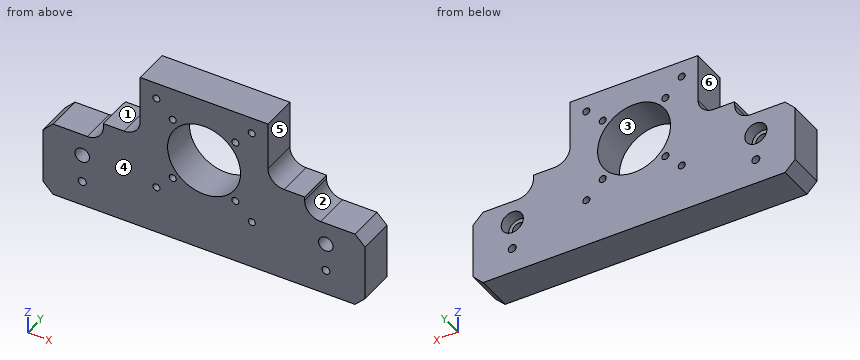
from build123d import *

# Parameters (mm, degrees)
F0_R           = 2
F0_W           = 63.5
F0_H           = 11.75
F0_R_2         = 1.75
F0_R_3         = 18.125
F1_DEPTH       = 18
F2_SIZE        = 5
F3_R           = 8
F4_D           = 7.2
F4_DEPTH       = 35
F4_CBORE_D     = 11
F4_CBORE_DEPTH = 6
F4_TIP         = 2.1630982285


with BuildPart() as f1:
    # F0 (on Front) → F1 (new body)
    with BuildSketch(Plane.XZ):
        Polygon((-80, -33.75), (80, -33.75), (80, 3.75), (50, 3.75), (50, 13.75), (31.75, 13.75), (31.75, -18), (-31.75, -18), (-31.75, 13.75), (-50, 13.75), (-50, 3.75), (-80, 3.75), align=None)
        with Locations((-60.5, -21.25)):
            Circle(F0_R, mode=Mode.SUBTRACT)
        with Locations((60.5, -21.25)):
            Circle(F0_R, mode=Mode.SUBTRACT)
        with Locations((0, 39.625)):
            Rectangle(F0_W, F0_H)
        with Locations((-23.6880771697, 37.4380771697)):
            Circle(F0_R_2, mode=Mode.SUBTRACT)
        with Locations((23.6880771697, 37.4380771697)):
            Circle(F0_R_2, mode=Mode.SUBTRACT)
        Polygon((31.75, 13.75), (31.75, 33.75), (-31.75, 33.75), (-31.75, 13.75), (-31.75, -18), (31.75, -18), align=None)
        with Locations((-23.6880771697, -9.9380771697)):
            Circle(F0_R_2, mode=Mode.SUBTRACT)
        with Locations((-15.5563491861, -1.8063491861)):
            Circle(F0_R_2, mode=Mode.SUBTRACT)
        with Locations((23.6880771697, -9.9380771697)):
            Circle(F0_R_2, mode=Mode.SUBTRACT)
        with Locations((15.5563491861, -1.8063491861)):
            Circle(F0_R_2, mode=Mode.SUBTRACT)
        with Locations((-15.5563491861, 29.3063491861)):
            Circle(F0_R_2, mode=Mode.SUBTRACT)
        with Locations((0, 13.75)):
            Circle(F0_R_3, mode=Mode.SUBTRACT)
        with Locations((15.5563491861, 29.3063491861)):
            Circle(F0_R_2, mode=Mode.SUBTRACT)
    extrude(amount=F1_DEPTH)

    # F2
    f2_edges = [f1.edges().sort_by_distance(p)[0] for p in [
        (-80, -9, -33.75),
        (80, -9, -33.75),
        (80, -9, 3.75),
        (-80, -9, 3.75),
    ]]
    chamfer(f2_edges, length=F2_SIZE)

    # F3
    f3_edges = [f1.edges().sort_by_distance(p)[0] for p in [
        (31.75, -9, 13.75),
        (-31.75, -9, 13.75),
        (50, -9, 3.75),
        (-50, -9, 3.75),
    ]]
    fillet(f3_edges, radius=F3_R)

    # F4
    with Locations(Plane(origin=(0, 0, 0), x_dir=(1, 0, 0), z_dir=(0, 1, 0))):
        with Locations((60.5, 7.25), (-60.5, 7.25)):
            CounterBoreHole(F4_D / 2, F4_CBORE_D / 2, F4_CBORE_DEPTH, depth=F4_DEPTH)
            with Locations((0, 0, -(F4_DEPTH + F4_TIP / 2))):  # 118° drill point
                Cone(0, F4_D / 2, F4_TIP, mode=Mode.SUBTRACT)


solid = f1.part
For this review, take the finished solid that the model builds, in its own axes (mm). Face numbers are marked on the shaded views. A direction names the side the tool comes from. Give positions to 0.01 mm unless a question says otherwise; leave off trailing zeros. Order: outer loops, then holes, each group sorted by start corner. A loop starts at its lowest first (then second) coordinate and runs counter-clockwise, first axis right, second up. Notation, with made-up numbers: (-17, 18.25) -> (25, 18.25) arc R22 cw to (25, 31.25) -> close; hole circle Ø2 at (55, 8). An arc over 180 degrees is marked (long way). Write item = value, one per line.
1) Insertion check: pin 1 (5 mm diameter, centred on x = 67.5, y = -8.5, fed in from +Z); pin 2 (2 mm diameter, centred on x = -15.56, z = -1.81, fed in from -Y); pin 3 (9 mm diameter, centred on x = -60.5, z = -7.25, fed in from +Y); pin 4 (8 mm diameter, centred on x = 43.5, y = -11, fed in from +Z). Each pin has a flat end and moves straight along its axis. Give the tip position at first contact, or say it passes through.
Findings:
pin_1 = 3.75
pin_2 = through
pin_3 = -6
pin_4 = 13.75
2) To check wall thickness, follow L1, parallel to Z at x = -60.5, y = -4.6; L2, parallel to X at y = -8.5, z = -7; L3, parallel to Z at x = -59, y = -10.5. State the ranges of each line that lie inside material, in increasing order. Write a range as from..to.
Findings:
L1 = -33.75..-23.25, -19.25..-12.75, -1.75..3.75
L2 = -80..-64.09, -56.91..56.91, 64.09..80
L3 = -33.75..-22.57, -19.93..-10.52, -3.98..3.75
3) We need section C-C, the plane y = -12.75. Count the separate pieces of the cut face and the enclosed holes in it, and give its area (3 significant figures).
Findings:
separate_pieces = 1
enclosed_holes = 13
area = 7,810 mm^2
4) We need section B-B, the plane z = -21.25. Give the boundary of the cut face in (x, y).
Findings:
outline = (-80, -18) -> (-62.5, -18) -> (-62.5, 0) -> (-80, 0) -> close; (-58.5, -18) -> (58.5, -18) -> (58.5, 0) -> (-58.5, 0) -> close; (62.5, -18) -> (80, -18) -> (80, 0) -> (62.5, 0) -> close
5) For the marked faces 4, 5 and 6, list the 3-axis set-ups (+Z, -Z, +X, -X, +Y, -Y) from which the entire face can be reached by the end or side of a thin tool; tool diameter is ignored.
Findings:
face_4 = +Z, -Z, +X, -X, -Y
face_5 = +Z, +X, +Y, -Y
face_6 = +Z, -X, +Y, -Y
6) We need section D-D, the plane x = -60.5. Give the boundary of the cut face in (y, z), and give its area (3 significant figures).
Findings:
outline = (-18, -33.75) -> (0, -33.75) -> (0, -23.25) -> (-18, -23.25) -> close; (-18, -19.25) -> (0, -19.25) -> (0, -12.75) -> (-6, -12.75) -> (-6, -10.85) -> (-18, -10.85) -> close; (-18, -3.65) -> (-6, -3.65) -> (-6, -1.75) -> (0, -1.75) -> (0, 3.75) -> (-18, 3.75) -> close
area = 451 mm^2
7) Draft analysis for pull direction X (two halves, no side actions). For the marked faces 1, 2 and 3, state which applies: pulls with the +X half, pulls with the -X half, needs draft (parallel to the pull), parting line crosses it, or undercut.
Findings:
face_1 = needs draft
face_2 = pulls with the +X half
face_3 = undercut
8) We need section A-A, the plane x = 0. Give the boundary of the cut face in (y, z) (3 decimals).
Findings:
outline = (-18, -33.75) -> (0, -33.75) -> (0, -4.375) -> (-18, -4.375) -> close; (-18, 31.875) -> (0, 31.875) -> (0, 45.5) -> (-18, 45.5) -> close
